Check sheet for the modelled part. Datum: model origin and axes. Units: mm. A direction names the side the tool comes from. Give positions to 0.01 mm unless a question says otherwise; leave off trailing zeros. Loops run counter-clockwise (first coordinate to the right, second up) from the corner with the lowest first, then second, coordinate; pieces in that order, holes last. Notation, with made-up numbers: M -29,-9 L -24,-9 A31 ccw -24,30 Z; hole C 65,-22.5 d10. An arc over 180 degrees is marked long. Write each question's results on one line, items separated by ' | '. Start each with the question number.
1. Go/stop test with flat-tipped pins: pin 1 (6 mm diameter, centred on y = 67.5, z = 4, fed in from +X); pin 2 (3 mm diameter, centred on x = 2.5, y = 31.5, fed in from -Z); pin 3 (10 mm diameter, centred on y = 62, z = -4.5, fed in from +X). Record where each tip stops, or that it passes through.
2. Sectioned sample at B-B on z = -2.5. Record the cut outline in (x, y).
3. Sectioned sample at C-C on y = 92. Record the cut outline in (x, z).
4. Sectioned sample at D-D on x = 7.25. Record the cut outline in (y, z), and give its area (3 significant figures).
5. Material ranges on line 1 along Y through (x, z) = (-5.5, 6); line 2 along Z through (x, y) = (-2.25, 42), recorded low to high.
6. Sectioned sample at A-A on x = 0. Record the cut outline in (y, z), and give its area (3 significant figures).
7. Tool access check on faces 1 (the flat face through (-7.465, 104.93, 4.391)), 2 (the flat face through (4, 100, -4)). Record the directions out of +Z, -Z, +X, -X, +Y, -Y that give a thin tool (end or side, any length) a straight path to the whole face; none if there is none.
Autodesk Inventor part; units mm, degrees
ref_plane "YZ Plane" through (0, 0, 0) normal (1, 0, 0) x (0, 1, 0)
ref_plane "XZ Plane" through (0, 0, 0) normal (0, 1, 0) x (-1, 0, 0)
ref_plane "XY Plane" through (0, 0, 0) normal (0, 0, 1) x (1, 0, 0)
sketch "Sketch1" plane through (0, 0, 0) normal (0, 1, 0) x (-1, 0, 0)
  circle A0 centre (0, 0) radius 5
  dimension "d0" = 10
extrude "Extrusion1" add sketch "Sketch1" along normal blind 100
thread "Thread1"
sketch "Sketch2" plane through (0, 100, 0) normal (0, 1, 0) x (1, 0, 0)
  circle A0 centre (0, 0) radius 5
  circle A1 centre (0, 0) radius 10 construction
  line L0 (-10, 0) -> (-5, 8.6603)
  line L1 (-5, 8.6603) -> (5, 8.6603)
  line L2 (5, 8.6603) -> (10, 0)
  line L3 (10, 0) -> (5, -8.6603)
  line L4 (5, -8.6603) -> (-5, -8.6603)
  line L5 (-5, -8.6603) -> (-10, 0)
  dimension "d5" = 20
extrude "Extrusion2" add sketch "Sketch2" along normal blind 10 contours A0 | L0 L1 L2 L3 L4 L5
properties part number "BoltA" material "Titanium"
Output values:
1) pin 1: x = 4.9 | pin 2: z = -4.9 | pin 3: x = 5
2) outline: M -8.56,100 L -4.33,100 L -4.33,0 L 4.33,0 L 4.33,100 L 8.56,100 L 8.56,110 L -8.56,110 Z
3) outline: C 0,0 d10
4) outline: M 100,-4.76 L 110,-4.76 L 110,4.76 L 100,4.76 Z | area: 95.3 mm2
5) line 1: 100 to 110 | line 2: -4.47 to 4.47
6) outline: M 0,-5 L 100,-5 L 100,-8.66 L 110,-8.66 L 110,8.66 L 100,8.66 L 100,5 L 0,5 Z | area: 1,170 mm2
7) face 1: +Z, -X, +Y, -Y | face 2: -Y
